Verification items for the finished model (mm, model axes). Face numbers are marked on the shaded views. A direction names the side the tool comes from. Give positions to 0.01 mm unless a question says otherwise; leave off trailing zeros. Write each loop counter-clockwise with the first axis right and the second up, starting at its lowest first coordinate (ties: lowest second). Pieces come first, ordered by that corner, then holes. Notation, with made-up numbers: (54.5, 83.25) -> (64.5, 83.25) arc R26 ccw to (64.5, 112.25) -> close; hole circle Ø3 at (30.25, -36.75). An arc over 180 degrees is marked (long way). Answer as CSV lines item,"result".
```python
from build123d import *

# Parameters (mm, degrees)
BOSS_EXTRUDE1_DEPTH     = 60
CUT_EXTRUDE2_DEPTH      = 10
SKETCH4_R               = 1.5
CUT_EXTRUDE3_DEPTH      = 145.308696897
CUT_EXTRUDE4_DEPTH      = 188.082869339
CUT_EXTRUDE4_DEPTH_BACK = 188.082869339
SKETCH6_W               = 5
SKETCH6_H               = 59
BOSS_EXTRUDE2_DEPTH     = 150
SKETCH7_R               = 7.5
SKETCH7_R_2             = 5.1
CUT_EXTRUDE5_DEPTH      = 148.732867027
SKETCH9_W               = 40
SKETCH9_H               = 10
CUT_EXTRUDE6_DEPTH      = 188.082869339
SKETCH11_W              = 10
SKETCH11_H              = 40
BOSS_EXTRUDE6_DEPTH     = 160
SKETCH13_W              = 40
SKETCH13_H              = 30
CUT_EXTRUDE7_DEPTH      = 156.32224567
BOSS_EXTRUDE7_DEPTH     = 60


with BuildPart() as part:
    # Sketch1 → Boss-Extrude1 (new, symmetric)
    with BuildSketch(Plane.YZ):
        Polygon((85, 50), (85, -50), (75, -50), (75, 40), (-75, 40), (-75, -50), (-85, -50), (-85, 50), align=None)
    extrude(amount=BOSS_EXTRUDE1_DEPTH, both=True)

    # Sketch3 → Cut-Extrude2 (cut)
    with BuildSketch(Plane.YZ.offset(60)):
        Polygon((-80, 45), (-80, -50), (-75, -50), (-75, 40), (75, 40), (75, -50), (80, -50), (80, 45), align=None)
    cut_extrude2 = extrude(amount=-CUT_EXTRUDE2_DEPTH, mode=Mode.SUBTRACT)

    # Mirror1: Cut-Extrude2 across plane
    add(cut_extrude2.mirror(Plane(origin=(0, 0, 0), x_dir=(0, 0, 1), z_dir=(1, 0, 0))), mode=Mode.SUBTRACT)

    # Sketch4 → Cut-Extrude3 (cut, through all)
    with BuildSketch(Plane.XY.offset(50)):
        with Locations((-35, 0)):
            Circle(SKETCH4_R)
        with Locations((35, 0)):
            Circle(SKETCH4_R)
        with Locations((-35, 60)):
            Circle(SKETCH4_R)
        with Locations((35, 60)):
            Circle(SKETCH4_R)
    extrude(amount=-CUT_EXTRUDE3_DEPTH, mode=Mode.SUBTRACT)

    # Sketch5 → Cut-Extrude4 (cut, two sides: drawn at the far end of the back side and taken through both)
    with BuildSketch(Plane(origin=(0, 85, 0), x_dir=(-1, 0, 0), z_dir=(0, 1, 0)).offset(-CUT_EXTRUDE4_DEPTH_BACK)):
        Polygon((45, 50), (-45, 50), (-45, -19), (20, -19), (45, -19), align=None)
    extrude(amount=CUT_EXTRUDE4_DEPTH + CUT_EXTRUDE4_DEPTH_BACK, mode=Mode.SUBTRACT)

    # Sketch6 → Boss-Extrude2 (add)
    with BuildSketch(Plane.XZ.offset(-75)):
        with Locations((-47.5, 10.5)):
            Rectangle(SKETCH6_W, SKETCH6_H)
        with Locations((47.5, 10.5)):
            Rectangle(SKETCH6_W, SKETCH6_H)
    extrude(amount=BOSS_EXTRUDE2_DEPTH)

    # Sketch7 → Cut-Extrude5 (cut, through all)
    with BuildSketch(Plane(origin=(-50, 0, 0), x_dir=(0, -1, 0), z_dir=(-1, 0, 0))):
        with Locations(Location((-50, 7, 0), (0, 0, 90))):
            Circle(SKETCH7_R)
        with Locations(Location((5, 8.5, 0), (0, 0, 90))):
            Circle(SKETCH7_R_2)
        with Locations(Location((50, 7, 0), (0, 0, 90))):
            Circle(SKETCH7_R)
    extrude(amount=-CUT_EXTRUDE5_DEPTH, mode=Mode.SUBTRACT)

    # Sketch9 → Cut-Extrude6 (cut, through all)
    with BuildSketch(Plane(origin=(0, 85, 0), x_dir=(-1, 0, 0), z_dir=(0, 1, 0))):
        with Locations((0, -45)):
            Rectangle(SKETCH9_W, SKETCH9_H)
    extrude(amount=-CUT_EXTRUDE6_DEPTH, mode=Mode.SUBTRACT)

    # Sketch11 → Boss-Extrude6 (add)
    with BuildSketch(Plane(origin=(0, -80, 0), x_dir=(-1, 0, 0), z_dir=(0, 1, 0))):
        with Locations((-55, -30)):
            Rectangle(SKETCH11_W, SKETCH11_H)
        with Locations((55, -30)):
            Rectangle(SKETCH11_W, SKETCH11_H)
    extrude(amount=BOSS_EXTRUDE6_DEPTH)

    # Sketch13 → Cut-Extrude7 (cut, through all)
    with BuildSketch(Plane(origin=(-60, 0, 0), x_dir=(0, -1, 0), z_dir=(-1, 0, 0))):
        with Locations((0, -35)):
            Rectangle(SKETCH13_W, SKETCH13_H)
    extrude(amount=-CUT_EXTRUDE7_DEPTH, mode=Mode.SUBTRACT)

    # Sketch14 → Boss-Extrude7 (add)
    with BuildSketch(Plane(origin=(0, 85, 0), x_dir=(-1, 0, 0), z_dir=(0, 1, 0))):
        Polygon((-45, 50), (-53, 50), (-53, -27), (-44.583399228, -27), (53, -27), (53, -19), (53, 50), (45, 50), (45, -19), (-45, -19), align=None)
    extrude(amount=BOSS_EXTRUDE7_DEPTH)


solid = part.part
```
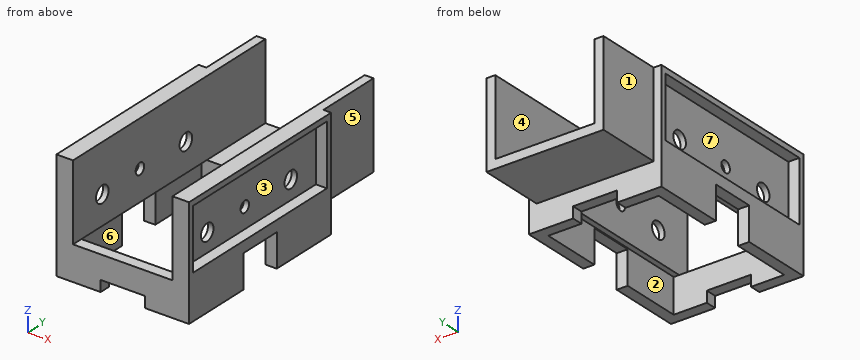
1) Section check B-B (z = 20). Record the boundary of the cut face in (x, y), and give its area (3 significant figures).
Reported:
outline,"(-60, -85) -> (-45, -85) -> (-45, 145) -> (-53, 145) -> (-53, 85) -> (-60, 85) -> (-60, 80) -> (-50, 80) -> (-50, -80) -> (-60, -80) -> close; (45, -85) -> (60, -85) -> (60, -80) -> (50, -80) -> (50, 80) -> (60, 80) -> (60, 85) -> (53, 85) -> (53, 145) -> (45, 145) -> close"
area,"2,860 mm²"
2) Draft check along X on the marked faces 5, 6 and 7. Enter one of: +X half, -X half, draft (parallel to the pull), parting line (faces both ways), or undercut.
Reported:
face 5,"+X half"
face 6,"undercut"
face 7,"-X half"
3) Section check C-C (x = 10.5). Record the boundary of the cut face in (y, z), and give its area (3 significant figures).
Reported:
outline,"(-85, -40) -> (-75, -40) -> (-75, -19) -> (-85, -19) -> close; (75, -40) -> (85, -40) -> (85, -27) -> (145, -27) -> (145, -19) -> (75, -19) -> close"
area,"900 mm²"
4) Scan lines: line 1 along Y through (x, z) = (6.5, -34); line 2 along X through (y, z) = (-12.5, 3); line 3 along X through (y, z) = (89.5, 27.5). Record each from-to range of solid material in increasing order.
Reported:
line 1,"-85 to -75, 75 to 85"
line 2,"-50 to -45, 45 to 50"
line 3,"-53 to -45, 45 to 53"
5) Section check A-A (y = 14). Record the boundary of the cut face in (x, z).
Reported:
outline,"(-60, -20) -> (-50, -20) -> (-50, -19) -> (-45, -19) -> (-45, 50) -> (-60, 50) -> (-60, 45) -> (-50, 45) -> (-50, -10) -> (-60, -10) -> close; (45, -19) -> (50, -19) -> (50, -20) -> (60, -20) -> (60, -10) -> (50, -10) -> (50, 45) -> (60, 45) -> (60, 50) -> (45, 50) -> close"
6) Tool access check on the marked faces 1, 2, 3 and 4. Record the directions out of +Z, -Z, +X, -X, +Y, -Y that give a thin tool (end or side, any length) a straight path to the whole face; none if there is none.
Reported:
face 1,"+Z, -Z, -X, +Y"
face 2,"-Z"
face 3,"+X"
face 4,"+Z, +Y, -Y"
7) Section check D-D (y = -50). Record the boundary of the cut face in (x, z).
Reported:
outline,"(-60, -50) -> (-50, -50) -> (-50, -19) -> (-45, -19) -> (-45, -0.5) -> (-50, -0.5) -> (-50, -10) -> (-60, -10) -> close; (-60, 45) -> (-50, 45) -> (-50, 14.5) -> (-45, 14.5) -> (-45, 50) -> (-60, 50) -> close; (45, -19) -> (50, -19) -> (50, -50) -> (60, -50) -> (60, -10) -> (50, -10) -> (50, -0.5) -> (45, -0.5) -> close; (45, 14.5) -> (50, 14.5) -> (50, 45) -> (60, 45) -> (60, 50) -> (45, 50) -> close"
8) Depth check by flat-ended pin: pin 1 (15.5 mm diameter, centred on y = 3, z = -34, fed in from +X); pin 2 (11 mm diameter, centred on x = -11.5, y = -78.5, fed in from +Z); pin 3 (3 mm diameter, centred on x = 56.5, z = -35, fed in from +Y); pin 4 (2 mm diameter, centred on y = -16.5, z = 29, fed in from -X). Enter the tip coordinate at first touch or a pass-through.
Reported:
pin 1,"through"
pin 2,"z = -19"
pin 3,"y = 85"
pin 4,"x = -50"
